```python
from build123d import *

# Parameters (mm, degrees)
SKETCH_1_R      = 2
SKETCH_1_R_2    = 1.55
SKETCH_1_R_3    = 1
SKETCH_1_R_4    = 2.5
EXTRUDE_1_DEPTH = 3


with BuildPart() as part:
    # 草图1 → 凸台-拉伸1 (new body)
    with BuildSketch(Plane.XY):
        with BuildLine():
            Line((-122.112109879, -103.385843426), (-122.112109879, -49.674836124))
            Line((-122.112109879, -49.674836124), (-84.112109879, -49.674836124))
            Line((-84.112109879, -49.674836124), (-84.112109879, -121.674836124))
            Line((-84.112109879, -121.674836124), (-103.900116719, -121.674836124))
            ThreePointArc((-103.900116719, -121.674836124), (0, -160), (103.900116719, -121.674836124))
            Line((103.900116719, -121.674836124), (84.112109879, -121.674836124))
            Line((84.112109879, -121.674836124), (84.112109879, -49.674836124))
            Line((84.112109879, -49.674836124), (122.112109879, -49.674836124))
            Line((122.112109879, -49.674836124), (122.112109879, -103.385843426))
            ThreePointArc((122.112109879, -103.385843426), (160, 0), (122.112109879, 103.385843426))
            Line((122.112109879, 103.385843426), (122.112109879, 49.674836124))
            Line((122.112109879, 49.674836124), (84.112109879, 49.674836124))
            Line((84.112109879, 49.674836124), (84.112109879, 121.674836124))
            Line((84.112109879, 121.674836124), (103.900116719, 121.674836124))
            ThreePointArc((103.900116719, 121.674836124), (0, 160), (-103.900116719, 121.674836124))
            Line((-103.900116719, 121.674836124), (-84.112109879, 121.674836124))
            Line((-84.112109879, 121.674836124), (-84.112109879, 49.674836124))
            Line((-84.112109879, 49.674836124), (-122.112109879, 49.674836124))
            Line((-122.112109879, 49.674836124), (-122.112109879, 103.385843426))
            ThreePointArc((-122.112109879, 103.385843426), (-160, 0), (-122.112109879, -103.385843426))
        make_face()
        with Locations((137.799674336, 18.195823561)):
            Circle(SKETCH_1_R, mode=Mode.SUBTRACT)
        with Locations((137.799674336, -18.804176439)):
            Circle(SKETCH_1_R, mode=Mode.SUBTRACT)
        with Locations((18.195823561, -137.799674336)):
            Circle(SKETCH_1_R, mode=Mode.SUBTRACT)
        with Locations((-18.804176439, -137.799674336)):
            Circle(SKETCH_1_R, mode=Mode.SUBTRACT)
        with Locations((-137.799674336, -18.195823561)):
            Circle(SKETCH_1_R, mode=Mode.SUBTRACT)
        with Locations((-137.799674336, 18.804176439)):
            Circle(SKETCH_1_R, mode=Mode.SUBTRACT)
        with Locations((-60.112109879, 93.674836124)):
            Circle(SKETCH_1_R_2, mode=Mode.SUBTRACT)
        with Locations((-60.112109879, 77.674836124)):
            Circle(SKETCH_1_R_2, mode=Mode.SUBTRACT)
        with Locations((-74.112109879, 93.674836124)):
            Circle(SKETCH_1_R_2, mode=Mode.SUBTRACT)
        with Locations((-74.112109879, 77.674836124)):
            Circle(SKETCH_1_R_2, mode=Mode.SUBTRACT)
        with Locations((0, -119)):
            Circle(SKETCH_1_R_3, mode=Mode.SUBTRACT)
        with Locations((0, -29)):
            Circle(SKETCH_1_R_3, mode=Mode.SUBTRACT)
        with Locations((-33.75, 9.85)):
            Circle(SKETCH_1_R_4, mode=Mode.SUBTRACT)
        with Locations((33.75, 9.85)):
            Circle(SKETCH_1_R_4, mode=Mode.SUBTRACT)
        with Locations((0, 41)):
            Circle(SKETCH_1_R_4, mode=Mode.SUBTRACT)
        with Locations((100.799676449, -37.721885932)):
            Circle(SKETCH_1_R, mode=Mode.SUBTRACT)
        with Locations((137.799674336, -37.734390952)):
            Circle(SKETCH_1_R, mode=Mode.SUBTRACT)
        with Locations((-137.799674336, -37.734390952)):
            Circle(SKETCH_1_R, mode=Mode.SUBTRACT)
        with Locations((-100.799676449, -37.721885932)):
            Circle(SKETCH_1_R, mode=Mode.SUBTRACT)
        with Locations((-18.804176439, 121.674836124)):
            Circle(SKETCH_1_R, mode=Mode.SUBTRACT)
        with Locations((18.195823561, 121.674836124)):
            Circle(SKETCH_1_R, mode=Mode.SUBTRACT)
        with Locations((74.112109879, 77.674836124)):
            Circle(SKETCH_1_R_2, mode=Mode.SUBTRACT)
        with Locations((74.112109879, 93.674836124)):
            Circle(SKETCH_1_R_2, mode=Mode.SUBTRACT)
        with Locations((60.112109879, 77.674836124)):
            Circle(SKETCH_1_R_2, mode=Mode.SUBTRACT)
        with Locations((60.112109879, 93.674836124)):
            Circle(SKETCH_1_R_2, mode=Mode.SUBTRACT)
        with Locations((60.112109879, -93.674836124)):
            Circle(SKETCH_1_R_2, mode=Mode.SUBTRACT)
        with Locations((60.112109879, -77.674836124)):
            Circle(SKETCH_1_R_2, mode=Mode.SUBTRACT)
        with Locations((74.112109879, -93.674836124)):
            Circle(SKETCH_1_R_2, mode=Mode.SUBTRACT)
        with Locations((74.112109879, -77.674836124)):
            Circle(SKETCH_1_R_2, mode=Mode.SUBTRACT)
        with Locations((-74.112109879, -77.674836124)):
            Circle(SKETCH_1_R_2, mode=Mode.SUBTRACT)
        with Locations((-74.112109879, -93.674836124)):
            Circle(SKETCH_1_R_2, mode=Mode.SUBTRACT)
        with Locations((-60.112109879, -77.674836124)):
            Circle(SKETCH_1_R_2, mode=Mode.SUBTRACT)
        with Locations((-60.112109879, -93.674836124)):
            Circle(SKETCH_1_R_2, mode=Mode.SUBTRACT)
    extrude(amount=EXTRUDE_1_DEPTH)


solid = part.part
```
Can you work these out from the model? Positions are in its coordinate system, mm. Give positions to 0.01 mm unless a question says otherwise; leave off trailing zeros. Write each loop counter-clockwise with the first axis right and the second up, starting at its lowest first coordinate (ties: lowest second). Pieces come first, ordered by that corner, then holes. Notation, with made-up numbers: (13.5, 17.5) - (39.5, 17.5) arc R35 cw to (39.5, 53.5) - close; hole circle Ø7 at (71.25, 34.25). An arc over 180 degrees is marked (long way). Write item = value, one per line. Start each with the question number.
1. Imagine slicing it at A-A (y = 68). Please give me the cut outline in (x, z).
2. Imagine slicing it at C-C (z = 1.9). Count the separate pieces of the cut face and the enclosed holes in it, and give its area (3 significant figures).
3. Imagine slicing it at B-B (y = -54). Please give me the cut outline in (x, z).
4. Please list where these lines run through material, in increasing order: line 1 (X direction, y = 54, z = 1.3); line 2 (X direction, y = -86, z = 0.95); line 3 (Y direction, x = -94, z = 1.55).
5. For pin 1 (5 mm diameter, centred on x = 74.11, y = 77.67, fed in from +Z); pin 2 (1.5 mm diameter, centred on y = 81, z = 1, fed in from +X), each with a flat end and sliding along its axis, tell me the tip position at first contact or that it passes through.
Worked answers:
q1.outline = (-144.83, 0) - (-122.11, 0) - (-122.11, 3) - (-144.83, 3) - close; (-84.11, 0) - (84.11, 0) - (84.11, 3) - (-84.11, 3) - close; (122.11, 0) - (144.83, 0) - (144.83, 3) - (122.11, 3) - close
q2.separate_pieces = 1
q2.enclosed_holes = 33
q2.area = 69,800 mm2
q3.outline = (-150.61, 0) - (-122.11, 0) - (-122.11, 3) - (-150.61, 3) - close; (-84.11, 0) - (84.11, 0) - (84.11, 3) - (-84.11, 3) - close; (122.11, 0) - (150.61, 0) - (150.61, 3) - (122.11, 3) - close
q4.line_1 = -150.61 to -122.11, -84.11 to 84.11, 122.11 to 150.61
q4.line_2 = -134.92 to -122.11, -84.11 to 84.11, 122.11 to 134.92
q4.line_3 = -129.48 to -121.67, -49.67 to 49.67, 121.67 to 129.48
q5.pin_1 = 3
q5.pin_2 = 138.42
